Geometry check sheet. Reference: drawing and pictorial views, mm from the part's lowest x, y, z. Give positions to 0.01 mm unless a question says otherwise; leave off trailing zeros. Write each loop counter-clockwise with the first axis right and the second up, starting at its lowest first coordinate (ties: lowest second). Pieces come first, ordered by that corner, then holes. Notation, with made-up numbers: M 88.5,80.5 L 126.5,80.5 A10 ccw 126.5,91.5 Z; hole C 62.5,81 d6. An arc over 180 degrees is marked long. Write item = value, one per line. Start each with the question number.
1) Scan lines: line 1 along X through (y, z) = (3.25, 20.5); line 2 along Z through (x, y) = (37.5, 6); line 3 along Y through (x, z) = (108.5, 28) (3 decimals). Record each from-to range of solid material in increasing order. Write a range as [from, to].
2) Mould release check, pull along Y, two halves, no side actions. Record for the marked faces 1, 2 and 3: released by +Y, released by -Y, zero draft, split by the parting line, or undercut.
3) Cross-section at C-C, the plane x = 27. Record the cut outline in (y, z).
4) Cross-section at D-D, the plane z = 36.5. Record the cut outline in (x, y) (3 decimals).
5) Go/stop test with flat-tipped pins: pin 1 (2 mm diameter, centred on y = 11.5, z = 36.5, fed in from -X); pin 2 (1.9 mm diameter, centred on x = 4.5, z = 40, fed in from +Y) (3 decimals); pin 3 (1.9 mm diameter, centred on y = 7, z = 17.5, fed in from -X); pin 4 (12.5 mm diameter, centred on x = 108, z = 19.5, fed in from -Y) (3 decimals). Record where each tip stops, or that it passes through.
6) Cross-section at A-A, the plane z = 21.5. Record the cut outline in (x, y) (3 decimals), plus the area to 3 significant figures.
7) Cross-section at B-B, the plane y = 6.35. Record the cut outline in (x, z).
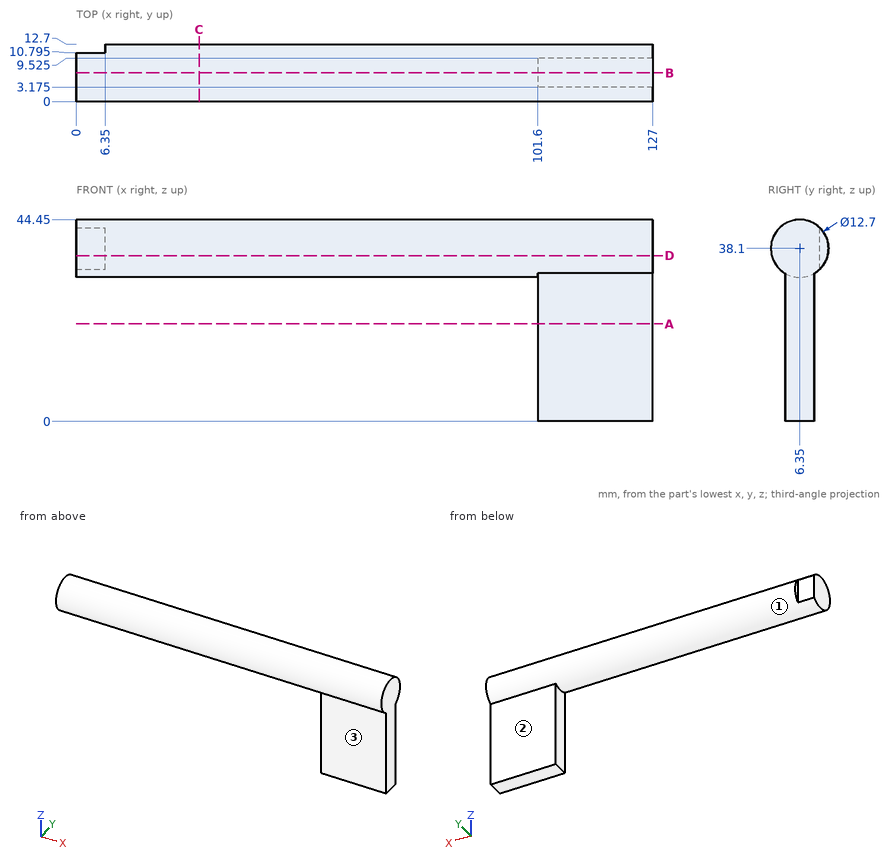
Reply:
q1.line_1 = [101.6, 127]
q1.line_2 = [31.76, 44.44]
q1.line_3 = [3.175, 9.525]
q2.face_1 = split by the parting line
q2.face_2 = released by +Y
q2.face_3 = released by -Y
q3.outline = C 6.35,38.1 d12.7
q4.outline = M 0,0.205 L 127,0.205 L 127,12.495 L 6.35,12.495 L 6.35,10.795 L 0,10.795 Z
q5.pin_1 = 0
q5.pin_2 = 10.795
q5.pin_3 = 101.6
q5.pin_4 = 3.175
q6.outline = M 101.6,3.175 L 127,3.175 L 127,9.525 L 101.6,9.525 Z
q6.area = 161 mm2
q7.outline = M 0,31.75 L 101.6,31.75 L 101.6,0 L 127,0 L 127,44.45 L 0,44.45 Z
